CAD build for the part. Positions are in the model's coordinates, mm. A direction names the side the tool comes from. Coordinates: 2 decimals unless noted, no trailing zeros. Write each loop counter-clockwise with the first axis right and the second up, starting at its lowest first coordinate (ties: lowest second). Pieces come first, ordered by that corner, then holes. Notation, with made-up numbers: (50, 10) - (82, 10) arc R19 ccw to (82, 17) - close; hole circle Ø9 at (14.5, 22). An arc over 180 degrees is marked (long way). Answer in a Markdown table with one row per item. Add a question column.
Q1. Band-saw the part on B-B (y = -87.5). List the corners of the cut face in (x, z).
Q2. Pin check, flat tips, straight feed: pin 1 (7.5 mm diameter, centred on x = 73.025, z = -126.483, fed in from -Y); pin 2 (4 mm diameter, centred on x = -188.5, z = 193.5, fed in from -Y); pin 3 (5 mm diameter, centred on x = -73.025, z = -126.483, fed in from +Y). Stop position of each tip, or through.
Q3. Two-plate mould, pull along X, no slides. Class faces 5 (the flat face through (-190, -99.06, 191)), 6 (the flat face through (-257, 0, -13)): +X half, -X half, draft (parallel to the pull), parting line (faces both ways), or undercut.
Q4. Drill centre lines: line 1 along X through (y, z) = (9, 0) (3 decimals); line 2 along X through (y, z) = (-100.55, 190.5); line 3 along X through (y, z) = (-100, 190). Where is each one in solid material? Low to high. Write a range as from..to.
Q5. 3-axis set-ups, long thin cutter, end or side, ignore diameter. For faces 1 (the flat face through (179.265, -50.089, -197.225)), 2 (the cylindrical face through (2.615, 6.261, 253.987)), 3 (the flat face through (179.265, -50.089, 197.225)), 4 (the cylindrical face through (179.73, -50.09, -179.48)): which of +Z, -Z, +X, -X, +Y, -Y reach the whole face in a straight line?
Q6. Band-saw the part on A-A (x = 0). List the corners of the cut face in (y, z).
Autodesk Inventor part; units mm, degrees
ref_plane "YZ Plane" through (0, 0, 0) normal (1, 0, 0) x (0, 1, 0)
ref_plane "XZ Plane" through (0, 0, 0) normal (0, 1, 0) x (-1, 0, 0)
ref_plane "XY Plane" through (0, 0, 0) normal (0, 0, 1) x (1, 0, 0)
sketch "Sketch1" plane through (0, 0, 0) normal (0, 1, 0) x (-1, 0, 0)
  circle A0 centre (0, 0) radius 254
  circle A1 centre (0, 0) radius 279.4
  line L0 (0, 279.4) -> (0, -279.4)
  line L1 (-279.4, 0) -> (279.4, 0)
  line L2 (197.5656, -197.5656) -> (-197.5656, 197.5656)
  line L3 (197.5656, 197.5656) -> (-197.5656, -197.5656)
  line L4 (206.5459, -188.5854) -> (-188.5854, 206.5459)
  line L5 (188.5854, -206.5459) -> (-206.5459, 188.5854)
  line L6 (188.5854, 206.5459) -> (-206.5459, -188.5854)
  line L7 (206.5459, 188.5854) -> (-188.5854, -206.5459)
  circle A2 centre (0, 0) radius 152.4
  circle A3 centre (0, 0) radius 101.6
  circle A4 centre (0, 0) radius 88.9
  circle A5 centre (0, 0) radius 139.7
  circle A6 centre (146.05, 0) radius 3.175
  circle A7 centre (73.025, 126.483) radius 3.175
  circle A8 centre (-73.025, 126.483) radius 3.175
  circle A9 centre (-146.05, 0) radius 3.175
  circle A10 centre (-73.025, -126.483) radius 3.175
  circle A11 centre (73.025, -126.483) radius 3.175
  circle A12 centre (95.25, 0) radius 3.175
  circle A13 centre (47.625, 82.4889) radius 3.175
  circle A14 centre (-47.625, 82.4889) radius 3.175
  circle A15 centre (-95.25, 0) radius 3.175
  circle A16 centre (-47.625, -82.4889) radius 3.175
  circle A17 centre (47.625, -82.4889) radius 3.175
  circle A18 centre (0, 0) radius 284.48
  point P0 (-170.4002, -188.3607)
  point P1 (-98.408, -116.3685)
  point P2 (98.408, -116.3685)
  point P3 (170.4002, -188.3607)
  point P4 (-188.3607, 170.4002)
  point P5 (-116.3685, 98.408)
  point P6 (-116.3685, -98.408)
  point P7 (-188.3607, -170.4002)
  point P8 (-170.4002, 188.3607)
  point P9 (170.4002, 188.3607)
  point P10 (98.408, 116.3685)
  point P11 (-98.408, 116.3685)
  point P12 (188.3607, -170.4002)
  point P13 (116.3685, -98.408)
  point P14 (116.3685, 98.408)
  point P15 (188.3607, 170.4002)
  point P16 (188.3812, 206.3417)
  point P17 (206.3417, 188.3812)
  point P18 (188.3812, -206.3417)
  point P19 (206.3417, -188.3812)
  point P20 (-206.3417, -188.3812)
  point P21 (-188.3812, -206.3417)
  point P22 (-188.3812, 206.3417)
  point P23 (-206.3417, 188.3812)
  dimension "d36" = 4
  dimension "d0" = 508
  dimension "d1" = 25.4
  dimension "d2" = 45
  dimension "d3" = 0
  dimension "d4" = 0
  dimension "d5" = 45
  dimension "d6" = 12.7
  dimension "d7" = 12.7
  dimension "d8" = 12.7
  dimension "d9" = 12.7
  dimension "d10" = 304.8
  dimension "d11" = 203.2
  dimension "d12" = 177.8
  dimension "d13" = 12.7
  dimension "d14" = 6.35
  dimension "d15" = 146.05
  dimension "d18" = 360
  dimension "d20" = 6.35
  dimension "d21" = 95.25
  dimension "d24" = 360
  dimension "d26" = 5.08
extrude "Extrusion1" add sketch "Sketch1" along normal blind 12.7 contours L1 A1 L4 A0 | A0 L7 A1 L1 | L7 A2 L3 A0 | A0 L3 A1 L7 | L4 A1 L2 A0 | A0 L2 A2 L4 | A2 L4 A5 L1 A6 | L1 A6 A5 L7 A2 | L3 A2 L6 A0 | A0 L6 A1 L3 | L7 A5 L3 A2 | L2 A1 L5 A0 | A0 L5 A2 L2 | A2 L2 A5 L4 | A0 L0 A1 L6 | L3 A5 L6 A2 | L5 A1 L0 A0 | A2 L5 A5 L2 | A0 L4 A1 L0 | L6 A5 L0 A2 | L0 A1 L7 A0 | A2 L0 A5 L5 | L4 A2 L2 A0 | A0 L2 A1 L4 | L0 A5 L4 A2 | L7 A1 L3 A0 | A0 L3 A2 L7 | A2 L7 A5 L0 | L2 A2 L5 A0 | A0 L5 A1 L2 | L4 A5 L2 A2 | L3 A1 L6 A0 | A0 L6 A2 L3 | A2 L3 A5 L7 | A0 L1 A1 L5 | L2 A5 L5 A2 | L6 A1 L1 A0 | A2 L6 A5 L3 | L5 A5 L1 A9 A2 | A2 L1 A9 A5 L6
extrude "Extrusion2" add sketch "Sketch1" against normal blind 101.6 contours A0 L3 A1 L7 | L4 A1 L2 A0 | A0 L6 A1 L3 | L2 A1 L5 A0 | A0 L2 A1 L4 | L7 A1 L3 A0 | A0 L5 A1 L2 | L3 A1 L6 A0
sketch "Sketch2" plane through (0, -101.6, 0) normal (0, -1, 0) x (1, 0, 0)
  circle A0 centre (-190.5, -190.5) radius 6.35
  line L0 (-188.3607, -170.4002) -> (-206.3417, -188.3812)
  arc A1 (-206.3417, -188.3812) -> (-188.3812, -206.3417) centre (0, 0) ccw
  dimension "d31" = 12.7
  dimension "d32" = 12.7
  dimension "d33" = 190.5
extrude "Extrusion3" cut sketch "Sketch2" against normal blind 2.54
pattern_circular "Circular Pattern1" count 4 over 360 about axis through (0, 0, 0) along (0, 1, 0) of "Extrusion3"
properties part number "Lazy suzan lower frame"
Checked values:
| question | item | result |
|---|---|---|
| 1 | outline | (-206.34, -188.38) arc R279.4 ccw to (-188.38, -206.34) - (-170.4, -188.36) arc R254 cw to (-188.36, -170.4) - close; (-206.34, 188.38) - (-188.36, 170.4) arc R254 cw to (-170.4, 188.36) - (-188.38, 206.34) arc R279.4 ccw to start; (170.4, -188.36) - (188.38, -206.34) arc R279.4 ccw to (206.34, -188.38) - (188.36, -170.4) arc R254 cw to start; (170.4, 188.36) arc R254 cw to (188.36, 170.4) - (206.34, 188.38) arc R279.4 ccw to (188.38, 206.34) - close |
| 2 | pin 1 | stops at y = 0 |
| 2 | pin 2 | stops at y = -99.06 |
| 2 | pin 3 | passes through |
| 3 | face 5 | undercut |
| 3 | face 6 | draft |
| 4 | line 1 | x = -279.4..-254, -152.4..-149.225, -142.875..-139.7, 139.7..142.875, 149.225..152.4, 254..279.4 |
| 4 | line 2 | x = -204.39..-196.85, -184.15..-172.54, 172.54..184.15, 196.85..204.39 |
| 4 | line 3 | x = -204.85..-196.83, -184.17..-172.04, 172.04..184.17, 196.83..204.85 |
| 5 | face 1 | -Z, -Y |
| 5 | face 2 | +Y, -Y |
| 5 | face 3 | +Z, -Y |
| 5 | face 4 | -Y |
| 6 | outline | (0, -279.4) - (12.7, -279.4) - (12.7, -254) - (0, -254) - close; (0, -152.4) - (12.7, -152.4) - (12.7, -139.7) - (0, -139.7) - close; (0, 139.7) - (12.7, 139.7) - (12.7, 152.4) - (0, 152.4) - close; (0, 254) - (12.7, 254) - (12.7, 279.4) - (0, 279.4) - close |
